Check sheet for the modelled part. Datum: model origin and axes. Units: mm. A direction names the side the tool comes from. Coordinates: 2 decimals unless noted, no trailing zeros. Loops run counter-clockwise (first coordinate to the right, second up) from the corner with the lowest first, then second, coordinate; pieces in that order, holes last. Notation, with made-up numbers: (11.25, 58) - (54.25, 58) arc R24 cw to (54.25, 95) - close; hole circle Ø1 at (81, -13). An arc over 180 degrees is marked (long way). Use a Markdown table: item, result. Add a question column.
1) Go/stop test with flat-tipped pins: P1, Ø5, axis at x = -7.5, y = 22.5, coming from the -Z side; P2, Ø4, axis at y = 10.5, z = 20.5, coming from the -X side; P3, Ø11, axis at y = 6.5, z = -23.5, coming from the +X side. Record where each tip stops, or that it passes through.
2) Sectioned sample at B-B, the plane y = 3. Enter the section's corners in (x, z).
3) Sectioned sample at D-D, the plane z = 24.5. Enter the section's corners in (x, y).
4) Draft check along Z on faces 5 (the flat face through (0, 5, -32.5)), 6 (the cylindrical face through (-15.935, 9.616, 6.607)), 7 (the flat face through (0, 10, -24)), 8 (the cylindrical face through (12.1, 12.32, 9.28)). Enter one of: pulls with the +Z half, pulls with the -Z half, needs draft (parallel to the pull), parting line crosses it, or undercut.
5) Thickness scan on line 1 (Z direction, x = -0.5, y = 6.75); line 2 (Z direction, x = 0, y = 15); line 3 (X direction, y = 8.5, z = 12.5). Record the ranges inside material, lowest first.
6) Tool access check on faces 1 (the flat face through (5, 5, 25)), 2 (the flat face through (5, 5, -24)), 3 (the flat face through (-5, 5, -25)), 4 (the flat face through (-5, 5, 24)). Record the directions out of +Z, -Z, +X, -X, +Y, -Y that give a thin tool (end or side, any length) a straight path to the whole face; none if there is none.
Autodesk Inventor part; units mm, degrees
ref_plane "YZ Plane" through (0, 0, 0) normal (1, 0, 0) x (0, 1, 0)
ref_plane "XZ Plane" through (0, 0, 0) normal (0, 1, 0) x (-1, 0, 0)
ref_plane "XY Plane" through (0, 0, 0) normal (0, 0, 1) x (1, 0, 0)
sketch "Sketch1" plane through (0, 0, 0) normal (0, 1, 0) x (-1, 0, 0)
  circle A0 centre (0, 0) radius 15.25
  circle A1 centre (0, 0) radius 17.25
  line L0 (5, 32.5) -> (-5, 32.5)
  line L1 (-5, 32.5) -> (-5, -32.5)
  line L2 (-5, -32.5) -> (5, -32.5)
  line L3 (5, -32.5) -> (5, 32.5)
  point P0 (0, -32.5)
  point P1 (5, 0)
  point P2 (5, -16.5095)
  point P3 (-5, -16.5095)
  point P4 (-5, 16.5095)
  point P5 (5, 16.5095)
  dimension "d0" = 30.5
  dimension "d1" = 2
  dimension "d7" = 10
  dimension "d8" = 65
extrude "Extrusion1" add sketch "Sketch1" along normal blind 25 contours A0 L3 A1 | A0 L1 A1 L3 | L3 A1 L1 A0 | A0 L1 A1
chamfer "Chamfer1" distance 2 angle 70 1 edges at (17.25, 25, 0) measured on face at (-16.4162, 25, -1.3761)
extrude "Extrusion2" add sketch "Sketch1" along normal blind 10 contours A1 L1 L0 L3 | L3 L2 L1 A1
properties part number "Pope8697-StopperCutter_3DPrint"
Solved:
| question | item | result |
|---|---|---|
| 1 | P1 | stops at z = -15.8 |
| 1 | P2 | stops at x = -5 |
| 1 | P3 | stops at x = 5 |
| 2 | outline | (-5, -32.5) - (5, -32.5) - (5, -16.51) arc R17.25 ccw to (5, 16.51) - (5, 32.5) - (-5, 32.5) - (-5, 16.51) arc R17.25 ccw to (-5, -16.51) - close; hole circle Ø30.5 at (0, 0) |
| 3 | outline | (-5, 0) - (5, 0) - (5, 10) - (-5, 10) - close |
| 4 | face 5 | pulls with the -Z half |
| 4 | face 6 | parting line crosses it |
| 4 | face 7 | needs draft |
| 4 | face 8 | undercut |
| 5 | line 1 | z = -32.5 to -15.24, 15.24 to 32.5 |
| 5 | line 2 | z = -17.25 to -15.25, 15.25 to 17.25 |
| 5 | line 3 | x = -11.89 to -8.74, 8.74 to 11.89 |
| 6 | face 1 | +Z, +X, +Y, -Y |
| 6 | face 2 | -Z, +X, +Y, -Y |
| 6 | face 3 | -Z, -X, +Y, -Y |
| 6 | face 4 | +Z, -X, +Y, -Y |
